```python
from build123d import *

# Parameters (mm, degrees)
SKETCH009_W             = 84
SKETCH009_H             = 70
PAD002_DEPTH            = 2
SKETCH010_W             = 2
SKETCH010_H             = 7
PAD003_DEPTH            = 2
SKETCH012_W             = 8
SKETCH012_H             = 6.8
PAD004_DEPTH            = 4
SKETCH013_W             = 7
SKETCH013_H             = 6
PAD005_DEPTH            = 4
SKETCH011_W             = 8
SKETCH011_H             = 6.8
PAD006_DEPTH            = 4
SKETCH014_R             = 1.15
POCKET002_DEPTH         = 81.001
SKETCH016_R             = 1.15
POCKET003_DEPTH         = 8.501
SKETCH018_W             = 11.5
SKETCH018_H             = 11.5
POCKET004_DEPTH         = 5
POCKET005_DEPTH         = 5
POCKET006_DEPTH         = 5
SKETCH021_W             = 1
SKETCH021_H             = 7
PAD007_DEPTH            = 1
SKETCH022_W             = 9
SKETCH022_H             = 10
POCKET007_DEPTH         = 0.4
FILLET_R                = 3
BODY002_PITCH_ANGLE     = -90
BODY002_PLACEMENT_ANGLE = 90
PAD001_DEPTH            = 35
SKETCH007_W             = 11.5
SKETCH007_H             = 11.5
POCKET001_DEPTH         = 13
FILLET001_R             = 3
SKETCH025_W             = 6.5
SKETCH025_H             = 9
SKETCH025_W_2           = 9
SKETCH025_H_2           = 6.5
POCKET008_DEPTH         = 8


with BuildPart() as back:
    # Sketch009 → Pad002 (new body)
    with BuildSketch(Plane.XY):
        Rectangle(SKETCH009_W, SKETCH009_H)
    extrude(amount=PAD002_DEPTH)

    # Sketch010 (on Face6 of Pad002) → Pad003 (join)
    with BuildSketch(Plane.XY.offset(2)):
        with Locations((-38, -1)):
            Rectangle(SKETCH010_W, SKETCH010_H)
        Polygon((-21, 32), (39, 32), (39, -4), (37, -4), (37, 30), (-21, 30), align=None)
    extrude(amount=PAD003_DEPTH)

    # Sketch012 (on Face15 of Pad003) → Pad004 (join)
    with BuildSketch(Plane.YZ.offset(39)):
        with Locations((0, 5.4)):
            Rectangle(SKETCH012_W, SKETCH012_H)
    extrude(amount=-PAD004_DEPTH)

    # Sketch013 (on Face9 of Pad004) → Pad005 (join)
    with BuildSketch(Plane(origin=(-39, 0, 0), x_dir=(0, -1, 0), z_dir=(-1, 0, 0))):
        with Locations((1, 5)):
            Rectangle(SKETCH013_W, SKETCH013_H)
    extrude(amount=-PAD005_DEPTH)

    # Sketch011 (on Face16 of Pad003) → Pad006 (join)
    with BuildSketch(Plane(origin=(0, 32, 0), x_dir=(-1, 0, 0), z_dir=(0, 1, 0))):
        with Locations((-29, 5.4)):
            Rectangle(SKETCH011_W, SKETCH011_H)
        with Locations((14, 5.4)):
            Rectangle(SKETCH011_W, SKETCH011_H)
    extrude(amount=-PAD006_DEPTH)

    # Sketch014 (on Face44 of Pad006) → Pocket002 (cut, through all)
    with BuildSketch(Plane.YZ.offset(39)):
        with Locations((0, 5)):
            Circle(SKETCH014_R)
    extrude(amount=-POCKET002_DEPTH, mode=Mode.SUBTRACT)

    # Sketch016 → Pocket003 (cut, through all)
    with BuildSketch(Plane.XZ.offset(-26.5)):
        with Locations((-13, 5)):
            Circle(SKETCH016_R)
        with Locations((30, 5)):
            Circle(SKETCH016_R)
    extrude(amount=-POCKET003_DEPTH, mode=Mode.SUBTRACT)

    # Sketch018 (on Face5 of Pocket003) → Pocket004 (cut)
    with BuildSketch(Plane.XY.offset(2)):
        with Locations((0, 17.75)):
            Rectangle(SKETCH018_W, SKETCH018_H)
    extrude(amount=-POCKET004_DEPTH, mode=Mode.SUBTRACT)

    # Sketch019 (on Face31 of Pocket004) → Pocket005 (cut)
    with BuildSketch(Plane.XZ.offset(-28)):
        Polygon((29.125944, 9.042901), (33.258869, 4.499726), (33.258869, 9.042901), align=None)
    extrude(amount=-POCKET005_DEPTH, mode=Mode.SUBTRACT)

    # Sketch020 (on Face36 of Pocket005) → Pocket006 (cut)
    with BuildSketch(Plane(origin=(35, 0, 0), x_dir=(0, -1, 0), z_dir=(-1, 0, 0))):
        Polygon((2.77547, 8.938441), (6.386171, 3.079567), (6.386171, 8.938441), align=None)
    extrude(amount=-POCKET006_DEPTH, mode=Mode.SUBTRACT)

    # Sketch021 (on Face40 of Pocket006) → Pad007 (join)
    with BuildSketch(Plane.XY.offset(8)):
        with Locations((-38.5, -1)):
            Rectangle(SKETCH021_W, SKETCH021_H)
    extrude(amount=PAD007_DEPTH)

    # Sketch022 (on Face5 of Pocket005) → Pocket007 (cut)
    with BuildSketch(Plane.XY.offset(2)):
        with Locations((-30.3, 30)):
            Rectangle(SKETCH022_W, SKETCH022_H)
    extrude(amount=-POCKET007_DEPTH, mode=Mode.SUBTRACT)

    # Fillet
    fillet_edges = [back.edges().sort_by_distance(p)[0] for p in [
        (42, 35, 1),
        (-42, 35, 1),
    ]]
    fillet(fillet_edges, radius=FILLET_R)


with BuildPart() as back_1:
    # Body002 pitch: moved
    add(back.part.rotate(Axis((0, 0, 0), (0, 1, 0)), BODY002_PITCH_ANGLE))


with BuildPart() as back_2:
    # Body002 placement: moved
    add(back_1.part.rotate(Axis((0, 0, 0), (0, 0, 1)), BODY002_PLACEMENT_ANGLE))


with BuildPart() as curve:
    # Sketch006 → Pad001 (new body, symmetric)
    with BuildSketch(Plane(origin=(0, 0, 0), x_dir=(0, 0, -1), z_dir=(1, 0, 0))):
        with BuildLine():
            ThreePointArc((-42, 3.9), (0, 0.863666), (42, 3.9))
            Line((42, -0.1), (42, 3.9))
            Line((-42, -0.1), (42, -0.1))
            Line((-42, 3.9), (-42, -0.1))
        make_face()
    extrude(amount=PAD001_DEPTH, both=True)

    # Sketch007 (on Face3 of Pad001) → Pocket001 (cut)
    with BuildSketch(Plane.XZ.offset(0.1)):
        with Locations((-17.75, 0)):
            Rectangle(SKETCH007_W, SKETCH007_H)
    extrude(amount=-POCKET001_DEPTH, mode=Mode.SUBTRACT)

    # Fillet001
    fillet001_edges = [curve.edges().sort_by_distance(p)[0] for p in [
        (-35, 1.9, -42),
        (-35, 1.9, 42),
    ]]
    fillet(fillet001_edges, radius=FILLET001_R)

    # Boolean: union Back
    add(back_2.part)

    # Sketch025 (on Face32 of Boolean) → Pocket008 (cut, symmetric)
    with BuildSketch(Plane.XZ.offset(2)):
        with Locations((-28.75, 0)):
            Rectangle(SKETCH025_W, SKETCH025_H)
        with Locations((-15.55, 13.625)):
            Rectangle(SKETCH025_W_2, SKETCH025_H_2)
        with Locations((-2.05, 0)):
            Rectangle(SKETCH025_W, SKETCH025_H)
        with Locations((-15.55, -13.625)):
            Rectangle(SKETCH025_W_2, SKETCH025_H_2)
    extrude(amount=POCKET008_DEPTH, both=True, mode=Mode.SUBTRACT)


solid = curve.part
```
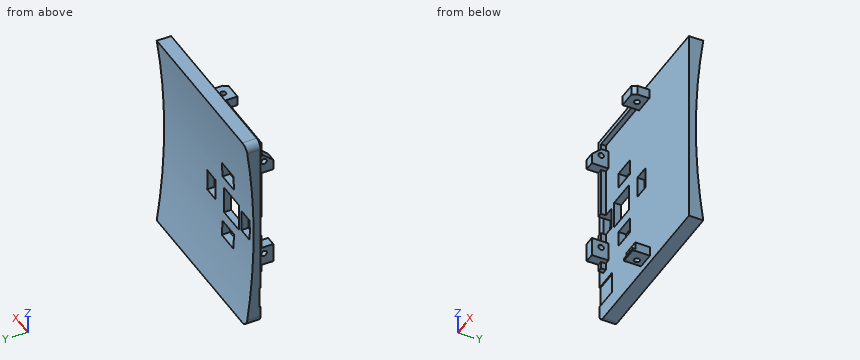
Model file for the job. Use its own axes, mm. Round coordinates to 2 decimals unless told otherwise and drop trailing zeros. Write each loop counter-clockwise with the first axis right and the second up, starting at its lowest first coordinate (ties: lowest second). Pieces come first, ordered by that corner, then holes. Notation, with made-up numbers: (43.25, -23.75) -> (94.25, -23.75) arc R24 cw to (94.25, 0.25) -> close; hole circle Ø1 at (49.5, 47). An arc over 180 degrees is marked (long way). Answer as CSV lines item,"result".
1. Slice it at C-C, the plane x = -9.5. List the corners of the cut face in (y, z), plus the area to 3 significant figures.
Resolved:
outline,"(-4, 37) -> (-2, 37) -> (-2, -42) -> (3.9, -42) arc R292 cw to (3.9, 42) -> (-2, 42) -> (-2, 39) -> (-4, 39) -> close"
area,"329 mm²"
2. Slice it at B-B, the plane z = -15.5. List the corners of the cut face in (x, y).
Resolved:
outline,"(-35, -2) -> (-32, -2) -> (-32, -8.8) -> (-28, -8.8) -> (-28, -2) -> (-20.05, -2) -> (-20.05, 1.28) -> (-35, 1.28) -> close; (-11.05, -2) -> (35, -2) -> (35, 1.28) -> (-11.05, 1.28) -> close"
3. Slice it at D-D, the plane z = 27.5. List the corners of the cut face in (x, y), plus the area to 3 significant figures.
Resolved:
outline,"(-35, -2) -> (-32, -2) -> (-32, -8.8) -> (-28, -8.8) -> (-28, -2) -> (35, -2) -> (35, 2.16) -> (-35, 2.16) -> close"
area,"319 mm²"
4. Slice it at A-A, the plane x = 0. List the corners of the cut face in (y, z), plus the area to 3 significant figures.
Resolved:
outline,"(-9, -39) -> (-6.15, -39) -> (-6.15, -35) -> (-8, -35) -> (-8, -38) -> (-9, -38) -> close; (-8.8, 35) -> (-6.15, 35) -> (-6.15, 39) -> (-8.8, 39) -> close; (-3.85, -39) -> (-2, -39) -> (-2, -42) -> (3.9, -42) arc R292 cw to (0.9, -4.5) -> (-2, -4.5) -> (-2, -35) -> (-3.85, -35) -> close; (-3.85, 35) -> (-2, 35) -> (-2, 4.5) -> (0.9, 4.5) arc R292 cw to (3.9, 42) -> (-2, 42) -> (-2, 39) -> (-3.85, 39) -> close"
area,"333 mm²"
5. Pin check, flat tips, straight feed: pin 1 Ø2 at (x, z) = (10, -15.5) entering from +Y; pin 2 Ø1.6 at (x, y) = (-16.5, -3) entering from -Z; pin 3 Ø0.9 at (x, z) = (2, -36.5) entering from -Y. Stop position of each tip, or through.
Resolved:
pin 1,"y = 1.33"
pin 2,"z = 37"
pin 3,"y = -8"
6. Drill centre lines: line 1 (X direction, y = 0.5, z = -15); line 2 (Y direction, x = -29, z = -13); line 3 (Y direction, x = -7.5, z = -10). Where is each one in solid material? Low to high.
Resolved:
line 1,"-35 to -20.05, -11.05 to 35"
line 2,"-8.8 to -6.15, -3.85 to 1.15"
line 3,"-2 to 1.03"
